Autodesk Inventor part; units mm, degrees
ref_plane "YZ Plane" through (0, 0, 0) normal (1, 0, 0) x (0, 1, 0)
ref_plane "XZ Plane" through (0, 0, 0) normal (0, 1, 0) x (-1, 0, 0)
ref_plane "XY Plane" through (0, 0, 0) normal (0, 0, 1) x (1, 0, 0)
sketch "Sketch1" plane through (0, 0, 0) normal (0, 0, 1) x (1, 0, 0)
  circle A0 centre (0, 0) radius 12.7
  dimension "d0" = 25.4
extrude "Extrusion1" add sketch "Sketch1" along normal blind 69.215
sketch "Sketch2" plane through (0, 0, 69.215) normal (0, 0, 1) x (1, 0, 0)
  circle A0 centre (0, 0) radius 12.7
  line L0 (0, 0) -> (-3.6945, 0)
  line L1 (1.19, 5.802) -> (1.19, 4.6114)
  arc A1 (-1.19, 4.6114) -> (1.19, 4.6114) centre (0, 0) ccw
  line L2 (-1.19, 4.6114) -> (-1.1912, 4.6114)
  line L3 (-1.1912, 4.6114) -> (-1.1912, 5.802)
  line L4 (-1.1912, 5.802) -> (1.19, 5.802)
extrude "Extrusion2" cut sketch "Sketch2" against normal blind 69.469 contours L1 A1 L3 L4
sketch "Sketch3" plane through (0, 0, 69.215) normal (0, 0, 1) x (1, 0, 0)
  line L0 (-1.1912, 4.6114) -> (-1.1912, 5.802)
  circle A0 centre (0, 0) radius 12.7
  line L1 (0, 0) -> (-3.175, 0)
  line L2 (-3.175, 12.2967) -> (-3.175, 9.1217)
  line L3 (-3.175, 9.1217) -> (3.175, 9.1217)
  line L4 (3.175, 9.1217) -> (3.175, 12.2967)
  dimension "d5" = 3.175
  dimension "d6" = 3.175
  dimension "d7" = 6.35
extrude "Extrusion3" cut sketch "Sketch3" against normal blind 69.469 contours L4 L3 L2 A0 picked at (-0.3561, 10.2995)
properties part number "winch insert" material "Aluminum 6061"
Verification items for the finished model (mm, model axes). A direction names the side the tool comes from. Coordinates: 2 decimals unless noted, no trailing zeros. Write each loop counter-clockwise with the first axis right and the second up, starting at its lowest first coordinate (ties: lowest second). Pieces come first, ordered by that corner, then holes. Notation, with made-up numbers: (70, 13) -> (109, 13) arc R21 ccw to (109, 27) -> close; hole circle Ø7 at (27, 2). An arc over 180 degrees is marked (long way). One line per item, written item: value. Start each with the question number.
Q1. Access from +Z, -Z, +X, -X, +Y, -Y to the whole of each face (thin tool, end or side, straight path). Record for faces 1 (the flat face through (0, 5.802, 35)), 2 (the flat face through (0, 9.122, 35)), 3 (the flat face through (0, -6, 0)).
Q2. Thickness scan on L1, parallel to X at y = 0, z = 54; L2, parallel to Y at x = -0.25, z = 45.5; L3, parallel to X at y = 1, z = 62.5. Record the ranges inside material, lowest first. Write a range as from..to.
Q3. Cross-section at D-D on y = -9.5. Enter the section's corners in (x, z) (3 decimals).
Q4. Cross-section at C-C on x = 0. Enter the section's corners in (y, z) (3 decimals).
Q5. Go/stop test with flat-tipped pins: P1, Ø1.6, axis at y = 10.5, z = 38.5, coming from the -X side; P2, Ø10, axis at x = -8, z = 48.5, coming from the -Y side; P3, Ø1.5, axis at x = -5, z = 13, coming from the +Y side; P4, Ø8.5, axis at x = 0, y = 0, coming from the +Z side. Record where each tip stops, or that it passes through.
Q6. Cross-section at A-A on y = 0. Enter the section's corners in (x, z) (3 decimals).
Q7. Mould release check, pull along X, two halves, no side actions. Record for faces 4 (the flat face through (-3.175, 11, 35)), 5 (the cylindrical face through (0.51, -12.69, 34.12)), 6 (the flat face through (0, -6, 69.215)): pulls with the +X half, pulls with the -X half, needs draft (parallel to the pull), parting line crosses it, or undercut.
Q8. Cross-section at B-B on z = 14. Enter the section's corners in (x, y) (3 decimals), and give its area (3 significant figures).
Checked values:
1. face 1: +Z, -Z
1. face 2: +Z, -Z, +Y
1. face 3: -Z, +X, -X, +Y, -Y
2. L1: x = -12.7..-4.76, 4.76..12.7
2. L2: y = -12.7..-4.76, 5.8..9.12
2. L3: x = -12.66..-4.66, 4.66..12.66
3. outline: (-8.429, 0) -> (8.429, 0) -> (8.429, 69.215) -> (-8.429, 69.215) -> close
4. outline: (-12.7, 0) -> (-4.762, 0) -> (-4.762, 69.215) -> (-12.7, 69.215) -> close; (5.802, 0) -> (9.122, 0) -> (9.122, 69.215) -> (5.802, 69.215) -> close
5. P1: stops at x = -8.2
5. P2: stops at y = -12.34
5. P3: stops at y = 11.97
5. P4: passes through
6. outline: (-12.7, 0) -> (-4.762, 0) -> (-4.762, 69.215) -> (-12.7, 69.215) -> close; (4.762, 0) -> (12.7, 0) -> (12.7, 69.215) -> (4.762, 69.215) -> close
7. face 4: undercut
7. face 5: parting line crosses it
7. face 6: needs draft
8. outline: (-3.175, 9.122) -> (-3.175, 12.297) arc R12.7 ccw (long way) to (3.175, 12.297) -> (3.175, 9.122) -> close; hole (-1.191, 5.802) -> (-1.19, 4.611) arc R4.762 ccw (long way) to (1.19, 4.611) -> (1.19, 5.802) -> close
8. area: 411 mm²
